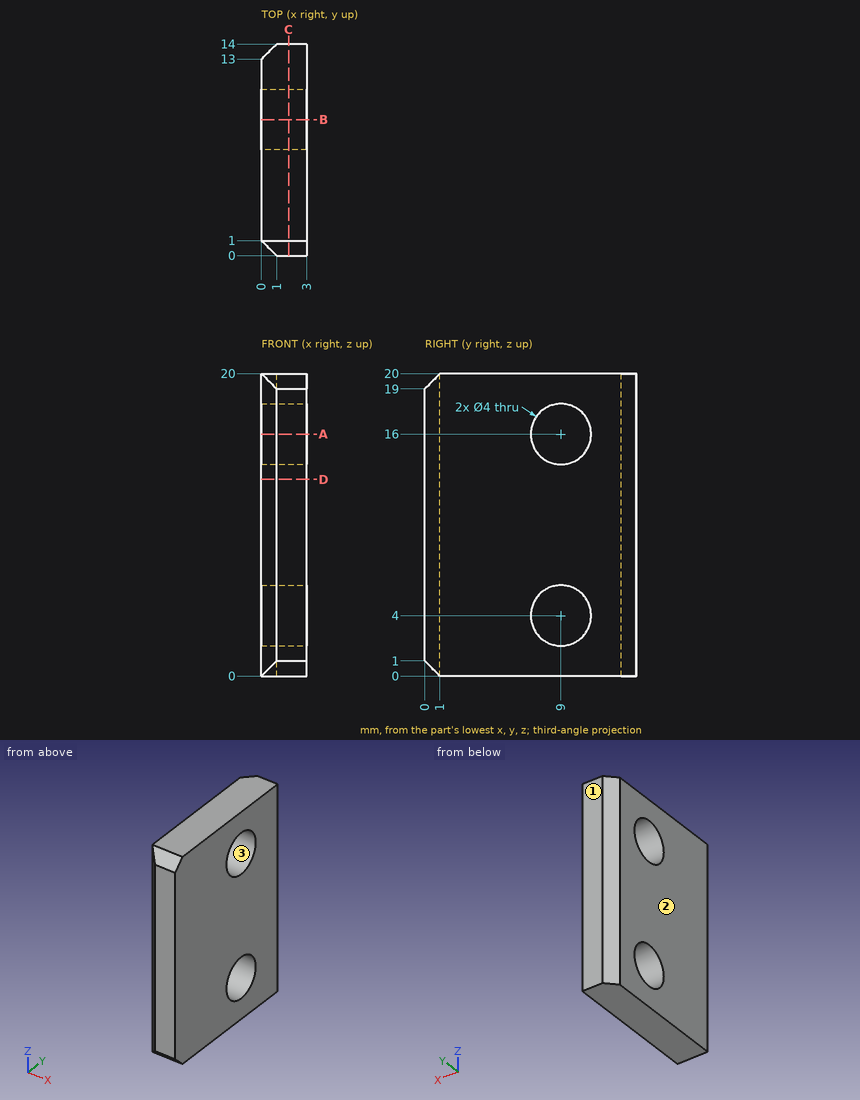
Could you check a few things on this drawing? It's one solid part, dimensions in mm from its lowest x, y, z. Coordinates: 2 decimals unless noted, no trailing zeros. Write each loop counter-clockwise with the first axis right and the second up, starting at its lowest first coordinate (ties: lowest second). Pieces come first, ordered by that corner, then holes. Notation, with made-up numbers: (20.25, 40.25) - (31.25, 40.25) arc R24 ccw to (31.25, 60.25) - close; hole circle Ø8 at (66.25, 66). An arc over 180 degrees is marked (long way). Use one line per item in the form item = value.
1) I need wall thicknesses on line 1 (Z direction, x = 1.55, y = 9); line 2 (Z direction, x = 1.55, y = 8.5); line 3 (Y direction, x = 1.05, z = 5.75). Which ranges of each line are inside material? Lowest first, please.
Solved:
line_1 = 0 to 2, 6 to 14, 18 to 20
line_2 = 0 to 2.06, 5.94 to 14.06, 17.94 to 20
line_3 = 0 to 8.03, 9.97 to 14
2) Suppose I cut it at C-C, the plane x = 1.8. Write out the boundary of the cut face in (y, z), plus the area to 3 significant figures.
Solved:
outline = (0, 1) - (1, 0) - (14, 0) - (14, 20) - (1, 20) - (0, 19) - close; hole circle Ø4 at (9, 4); hole circle Ø4 at (9, 16)
area = 254 mm2
3) Suppose I cut it at D-D, the plane z = 13. Write out the boundary of the cut face in (x, y), plus the area to 3 significant figures.
Solved:
outline = (0, 1) - (1, 0) - (3, 0) - (3, 14) - (1, 14) - (0, 13) - close
area = 41.0 mm2
4) Suppose I cut it at B-B, the plane y = 9. Write out the boundary of the cut face in (x, z), plus the area to 3 significant figures.
Solved:
outline = (0, 0) - (3, 0) - (3, 2) - (0, 2) - close; (0, 6) - (3, 6) - (3, 14) - (0, 14) - close; (0, 18) - (3, 18) - (3, 20) - (0, 20) - close
area = 36.0 mm2
5) Thinking about a two-plate mould opening in Y: for the marked faces 1, 2 and 3, which applies, released by +Y, released by -Y, zero draft, split by the parting line, or undercut?
Solved:
face_1 = released by +Y
face_2 = zero draft
face_3 = undercut
6) Suppose I cut it at A-A, the plane z = 16. Write out the boundary of the cut face in (x, y).
Solved:
outline = (0, 1) - (1, 0) - (3, 0) - (3, 7) - (0, 7) - close; (0, 11) - (3, 11) - (3, 14) - (1, 14) - (0, 13) - close
